Autodesk Fusion 360 part; units mm, degrees
sketch "Sketch1" plane through (0, 0, 0) normal (0, 1, 0) x (1, 0, 0)
  circle A0 centre (0, 0) radius 90 construction
  line L0 (-81.9196, 14.4446) -> (-88.6327, 15.6283)
  line L1 (-88.6327, 15.6283) -> (-83.1834, 0)
  line L2 (-90, 0) -> (-81.9196, -14.4446)
  line L3 (-83.1834, 0) -> (-90, 0)
  line L4 (-88.6327, -15.6283) -> (-78.1668, -28.4504)
  line L5 (-81.9196, -14.4446) -> (-88.6327, -15.6283)
  line L6 (-84.5723, -30.7818) -> (-72.0389, -41.5917)
  line L7 (-78.1668, -28.4504) -> (-84.5723, -30.7818)
  line L8 (-77.9423, -45) -> (-63.7222, -53.4693)
  line L9 (-72.0389, -41.5917) -> (-77.9423, -45)
  line L10 (-68.944, -57.8509) -> (-53.4693, -63.7222)
  line L11 (-63.7222, -53.4693) -> (-68.944, -57.8509)
  line L12 (-57.8509, -68.944) -> (-41.5917, -72.0389)
  line L13 (-53.4693, -63.7222) -> (-57.8509, -68.944)
  line L14 (-45, -77.9423) -> (-28.4504, -78.1668)
  line L15 (-41.5917, -72.0389) -> (-45, -77.9423)
  line L16 (-30.7818, -84.5723) -> (-14.4446, -81.9196)
  line L17 (-28.4504, -78.1668) -> (-30.7818, -84.5723)
  line L18 (-15.6283, -88.6327) -> (0, -83.1834)
  line L19 (-14.4446, -81.9196) -> (-15.6283, -88.6327)
  line L20 (0, -90) -> (14.4446, -81.9196)
  line L21 (0, -83.1834) -> (0, -90)
  line L22 (15.6283, -88.6327) -> (28.4504, -78.1668)
  line L23 (14.4446, -81.9196) -> (15.6283, -88.6327)
  line L24 (30.7818, -84.5723) -> (41.5917, -72.0389)
  line L25 (28.4504, -78.1668) -> (30.7818, -84.5723)
  line L26 (45, -77.9423) -> (53.4693, -63.7222)
  line L27 (41.5917, -72.0389) -> (45, -77.9423)
  line L28 (57.8509, -68.944) -> (63.7222, -53.4693)
  line L29 (53.4693, -63.7222) -> (57.8509, -68.944)
  line L30 (68.944, -57.8509) -> (72.0389, -41.5917)
  line L31 (63.7222, -53.4693) -> (68.944, -57.8509)
  line L32 (77.9423, -45) -> (78.1668, -28.4504)
  line L33 (72.0389, -41.5917) -> (77.9423, -45)
  line L34 (84.5723, -30.7818) -> (81.9196, -14.4446)
  line L35 (78.1668, -28.4504) -> (84.5723, -30.7818)
  line L36 (88.6327, -15.6283) -> (83.1834, 0)
  line L37 (81.9196, -14.4446) -> (88.6327, -15.6283)
  line L38 (90, 0) -> (81.9196, 14.4446)
  line L39 (83.1834, 0) -> (90, 0)
  line L40 (88.6327, 15.6283) -> (78.1668, 28.4504)
  line L41 (81.9196, 14.4446) -> (88.6327, 15.6283)
  line L42 (84.5723, 30.7818) -> (72.0389, 41.5917)
  line L43 (78.1668, 28.4504) -> (84.5723, 30.7818)
  line L44 (77.9423, 45) -> (63.7222, 53.4693)
  line L45 (72.0389, 41.5917) -> (77.9423, 45)
  line L46 (68.944, 57.8509) -> (53.4693, 63.7222)
  line L47 (63.7222, 53.4693) -> (68.944, 57.8509)
  line L48 (57.8509, 68.944) -> (41.5917, 72.0389)
  line L49 (53.4693, 63.7222) -> (57.8509, 68.944)
  line L50 (45, 77.9423) -> (28.4504, 78.1668)
  line L51 (41.5917, 72.0389) -> (45, 77.9423)
  line L52 (30.7818, 84.5723) -> (14.4446, 81.9196)
  line L53 (28.4504, 78.1668) -> (30.7818, 84.5723)
  line L54 (15.6283, 88.6327) -> (0, 83.1834)
  line L55 (14.4446, 81.9196) -> (15.6283, 88.6327)
  line L56 (0, 90) -> (-14.4446, 81.9196)
  line L57 (0, 83.1834) -> (0, 90)
  line L58 (-15.6283, 88.6327) -> (-28.4504, 78.1668)
  line L59 (-14.4446, 81.9196) -> (-15.6283, 88.6327)
  line L60 (-30.7818, 84.5723) -> (-41.5917, 72.0389)
  line L61 (-28.4504, 78.1668) -> (-30.7818, 84.5723)
  line L62 (-45, 77.9423) -> (-53.4693, 63.7222)
  line L63 (-41.5917, 72.0389) -> (-45, 77.9423)
  line L64 (-57.8509, 68.944) -> (-63.7222, 53.4693)
  line L65 (-53.4693, 63.7222) -> (-57.8509, 68.944)
  line L66 (-68.944, 57.8509) -> (-72.0389, 41.5917)
  line L67 (-63.7222, 53.4693) -> (-68.944, 57.8509)
  line L68 (-77.9423, 45) -> (-78.1668, 28.4504)
  line L69 (-72.0389, 41.5917) -> (-77.9423, 45)
  line L70 (-84.5723, 30.7818) -> (-81.9196, 14.4446)
  line L71 (-78.1668, 28.4504) -> (-84.5723, 30.7818)
  circle A1 centre (0, 0) radius 7.9405
  dimension "d1" = 180
  dimension "d5" = 15.881
extrude "Extrude1" add sketch "Sketch1" along normal blind 2.32
sketch "Sketch2" plane through (0, 2.32, 0) normal (0, 1, 0) x (-1, 0, 0)
  circle A0 centre (0, 0) radius 7.9405
  line L0 (78.1668, -28.4504) -> (84.5723, -30.7818)
  line L1 (84.5723, -30.7818) -> (81.9196, -14.4446)
  line L2 (81.9196, -14.4446) -> (88.6327, -15.6283)
  line L3 (88.6327, -15.6283) -> (83.1834, 0)
  line L4 (83.1834, 0) -> (90, 0)
  line L5 (90, 0) -> (81.9196, 14.4446)
  line L6 (81.9196, 14.4446) -> (88.6327, 15.6283)
  line L7 (88.6327, 15.6283) -> (78.1668, 28.4504)
  line L8 (78.1668, 28.4504) -> (84.5723, 30.7818)
  line L9 (84.5723, 30.7818) -> (72.0389, 41.5917)
  line L10 (72.0389, 41.5917) -> (77.9423, 45)
  line L11 (77.9423, 45) -> (63.7222, 53.4693)
  line L12 (63.7222, 53.4693) -> (68.944, 57.8509)
  line L13 (68.944, 57.8509) -> (53.4693, 63.7222)
  line L14 (53.4693, 63.7222) -> (57.8509, 68.944)
  line L15 (57.8509, 68.944) -> (41.5917, 72.0389)
  line L16 (41.5917, 72.0389) -> (45, 77.9423)
  line L17 (45, 77.9423) -> (28.4504, 78.1668)
  line L18 (28.4504, 78.1668) -> (30.7818, 84.5723)
  line L19 (30.7818, 84.5723) -> (14.4446, 81.9196)
  line L20 (14.4446, 81.9196) -> (15.6283, 88.6327)
  line L21 (15.6283, 88.6327) -> (0, 83.1834)
  line L22 (0, 83.1834) -> (0, 90)
  line L23 (0, 90) -> (-14.4446, 81.9196)
  line L24 (-14.4446, 81.9196) -> (-15.6283, 88.6327)
  line L25 (-15.6283, 88.6327) -> (-28.4504, 78.1668)
  line L26 (-28.4504, 78.1668) -> (-30.7818, 84.5723)
  line L27 (-30.7818, 84.5723) -> (-41.5917, 72.0389)
  line L28 (-41.5917, 72.0389) -> (-45, 77.9423)
  line L29 (-45, 77.9423) -> (-53.4693, 63.7222)
  line L30 (-53.4693, 63.7222) -> (-57.8509, 68.944)
  line L31 (-57.8509, 68.944) -> (-63.7222, 53.4693)
  line L32 (-63.7222, 53.4693) -> (-68.944, 57.8509)
  line L33 (-68.944, 57.8509) -> (-72.0389, 41.5917)
  line L34 (-72.0389, 41.5917) -> (-77.9423, 45)
  line L35 (-77.9423, 45) -> (-78.1668, 28.4504)
  line L36 (-78.1668, 28.4504) -> (-84.5723, 30.7818)
  line L37 (-84.5723, 30.7818) -> (-81.9196, 14.4446)
  line L38 (-81.9196, 14.4446) -> (-88.6327, 15.6283)
  line L39 (-88.6327, 15.6283) -> (-83.1834, 0)
  line L40 (-83.1834, 0) -> (-90, 0)
  line L41 (-90, 0) -> (-81.9196, -14.4446)
  line L42 (-81.9196, -14.4446) -> (-88.6327, -15.6283)
  line L43 (-88.6327, -15.6283) -> (-78.1668, -28.4504)
  line L44 (-78.1668, -28.4504) -> (-84.5723, -30.7818)
  line L45 (-84.5723, -30.7818) -> (-72.0389, -41.5917)
  line L46 (-72.0389, -41.5917) -> (-77.9423, -45)
  line L47 (-77.9423, -45) -> (-63.7222, -53.4693)
  line L48 (-63.7222, -53.4693) -> (-68.944, -57.8509)
  line L49 (-68.944, -57.8509) -> (-53.4693, -63.7222)
  line L50 (-53.4693, -63.7222) -> (-57.8509, -68.944)
  line L51 (-57.8509, -68.944) -> (-41.5917, -72.0389)
  line L52 (-41.5917, -72.0389) -> (-45, -77.9423)
  line L53 (-45, -77.9423) -> (-28.4504, -78.1668)
  line L54 (-28.4504, -78.1668) -> (-30.7818, -84.5723)
  line L55 (-30.7818, -84.5723) -> (-14.4446, -81.9196)
  line L56 (-14.4446, -81.9196) -> (-15.6283, -88.6327)
  line L57 (-15.6283, -88.6327) -> (0, -83.1834)
  line L58 (0, -83.1834) -> (0, -90)
  line L59 (0, -90) -> (14.4446, -81.9196)
  line L60 (14.4446, -81.9196) -> (15.6283, -88.6327)
  line L61 (15.6283, -88.6327) -> (28.4504, -78.1668)
  line L62 (28.4504, -78.1668) -> (30.7818, -84.5723)
  line L63 (30.7818, -84.5723) -> (41.5917, -72.0389)
  line L64 (41.5917, -72.0389) -> (45, -77.9423)
  line L65 (45, -77.9423) -> (53.4693, -63.7222)
  line L66 (53.4693, -63.7222) -> (57.8509, -68.944)
  line L67 (57.8509, -68.944) -> (63.7222, -53.4693)
  line L68 (63.7222, -53.4693) -> (68.944, -57.8509)
  line L69 (68.944, -57.8509) -> (72.0389, -41.5917)
  line L70 (72.0389, -41.5917) -> (77.9423, -45)
  line L71 (77.9423, -45) -> (78.1668, -28.4504)
  circle A1 centre (0, -50) radius 3.5
  circle A2 centre (47.5528, -15.4508) radius 3.5
  circle A3 centre (29.3893, 40.4508) radius 3.5
  circle A4 centre (-29.3893, 40.4508) radius 3.5
  circle A5 centre (-47.5528, -15.4508) radius 3.5
  dimension "d8" = 7
  dimension "d10" = 360
extrude "Extrude2" cut sketch "Sketch2" against normal blind 30 contours A1 | A2 | A3 | A4 | A5
For this review, take the finished solid that the model builds, in its own axes (mm). A direction names the side the tool comes from. Coordinates: 2 decimals unless noted, no trailing zeros. Loops run counter-clockwise (first coordinate to the right, second up) from the corner with the lowest first, then second, coordinate; pieces in that order, holes last. Notation, with made-up numbers: (45, 65.25) - (72, 65.25) arc R18 ccw to (72, 99.25) - close; hole circle Ø6 at (46, -3.75). An arc over 180 degrees is marked (long way). Return JSON: item names as keys, results as strings.
Item 1: Mouldability with a two-part tool opening along Z and no side actions: class faces 1 (the flat face through (-1, 0, 19)), 2 (the flat face through (83.473, 1.144, -21.95)), 3 (the flat face through (-21.95, 1.144, -83.473)) as pulls with the +Z half, pulls with the -Z half, needs draft (parallel to the pull), parting line crosses it, or undercut.
Determined:
{"face 1": "needs draft", "face 2": "undercut", "face 3": "pulls with the -Z half"}
Item 2: Take a section at A-A (x = -75.5). Give the boundary of the cut face in (y, z).
Determined:
{"outline": "(0, -43.59) - (2.32, -43.59) - (2.32, 38.61) - (0, 38.61) - close; (0, 43.59) - (2.32, 43.59) - (2.32, 46.45) - (0, 46.45) - close"}
Item 3: For line 1 (X direction, y = 1.4, z = -13); line 2 (X direction, y = 0.75, z = -51); line 3 (X direction, y = 1.25, z = 55.5), list the stretches that pass through material, from the lowest coordinate up.
Determined:
{"line 1": "x = -87.72 to -50.05, -45.05 to 45.05, 50.05 to 82.73", "line 2": "x = -70.25 to -3.35, 3.35 to 67.87", "line 3": "x = -66.14 to 62.95, 66.14 to 69.39"}
Item 4: Take a section at D-D (x = 10). Give the boundary of the cut face in (y, z), then the cut area to 3 significant figures.
Determined:
{"outline": "(0, -86.67) - (2.32, -86.67) - (2.32, 84.41) - (0, 84.41) - close", "area": "397 mm2"}
Item 5: Take a section at C-C (y = 1.85). State how many separate pieces and enclosed holes the cut face has, then the cut area to 3 significant figures.
Determined:
{"separate pieces": "1", "enclosed holes": "6", "area": "23,000 mm2"}
Item 6: For faces 4 (the flat face through (-78.393, 1.144, 36.111)), 5 (the flat face through (55.63, 1.14, 66.3)), 6 (the flat face through (55.63, 1.14, -66.3)), 7 (the cylindrical face through (-32.73, 1.18, 41.5)), 8 (the flat face through (-55.63, 1.14, -66.3)), list the 3-axis set-ups (+Z, -Z, +X, -X, +Y, -Y) from which the entire face can be reached by the end or side of a thin tool; tool diameter is ignored.
Determined:
{"face 4": "-X, +Y, -Y", "face 5": "+Z, +Y, -Y", "face 6": "+X, +Y, -Y", "face 7": "+Y, -Y", "face 8": "-Z, +Y, -Y"}
Item 7: Insertion check: pin 1 (1.2 mm diameter, centred on x = -87.5, y = 1, fed in from -Z); pin 2 (1.2 mm diameter, centred on y = 1.5, z = -87.5, fed in from +X); pin 3 (0.7 mm diameter, centred on x = 87, y = 1, fed in from +Z); pin 4 (4 mm diameter, centred on x = -47.55, z = -15.45, fed in from +Y). Each pin has a flat end and moves straight along its axis. Give the tip position at first contact, or say it passes through.
Determined:
{"pin 1": "stops at z = -15.53", "pin 2": "stops at x = 15.53", "pin 3": "stops at z = 15.4", "pin 4": "passes through"}
Item 8: Take a section at B-B (z = 4). Give the boundary of the cut face in (x, y).
Determined:
{"outline": "(-87.76, 0) - (-6.86, 0) - (-6.86, 2.32) - (-87.76, 2.32) - close; (6.86, 0) - (84.58, 0) - (84.58, 2.32) - (6.86, 2.32) - close"}
